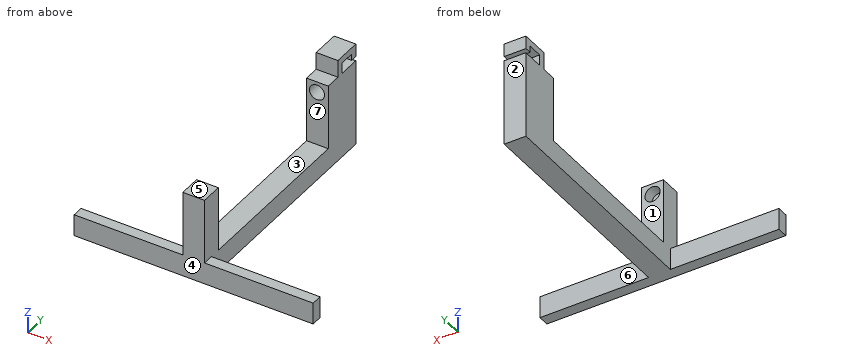
```python
from build123d import *

# Parameters (mm, degrees)
SKICA1_W                      = 10
SKICA1_H                      = 10
P_IDAT_VYSUNUT_M1_DEPTH       = 10
SKICA2_R                      = 3.5
ODEBRAT_VYSUNUT_M1_DEPTH      = 5
SKICA6_W                      = 10
SKICA6_H                      = 10
P_IDAT_VYSUNUT_M9_DEPTH       = 30
SKICA7_W                      = 10
SKICA7_H                      = 10
P_IDAT_VYSUNUT_M11_DEPTH      = 100
SKICA8_W                      = 10
SKICA8_H                      = 10
P_IDAT_VYSUNUT_M12_DEPTH      = 30
SKICA9_W                      = 10
SKICA9_H                      = 10
P_IDAT_VYSUNUT_M13_DEPTH      = 10
SKICA10_R                     = 3.5
ODEBRAT_VYSUNUT_M2_DEPTH      = 10
SKICA20_W                     = 10
SKICA20_H                     = 10
P_IDAT_VYSUNUT_M21_DEPTH      = 20
P_IDAT_VYSUNUT_M22_DEPTH      = 50
P_IDAT_VYSUNUT_M22_DEPTH_BACK = 60
SKICA11_W                     = 10
SKICA11_H                     = 5
SKICA10_2_R                   = 3.5
ODEBRAT_VYSUNUT_M7_DEPTH      = 15
SKICA21_W                     = 10
SKICA21_H                     = 3
P_IDAT_VYSUNUT_M24_DEPTH      = 8
SKICA22_W                     = 10
SKICA22_H                     = 3
P_IDAT_VYSUNUT_M25_DEPTH      = 10
SKICA23_W                     = 10
SKICA23_H                     = 3
P_IDAT_VYSUNUT_M26_DEPTH      = 3


with BuildPart() as part:
    # Skica1 → P_idat vysunut_m1 (new body)
    with BuildSketch(Plane.XY):
        with Locations((5, 5)):
            Rectangle(SKICA1_W, SKICA1_H)
    extrude(amount=P_IDAT_VYSUNUT_M1_DEPTH)

    # Skica2 → Odebrat vysunut_m1 (cut)
    with BuildSketch(Plane(origin=(0, 10, 0), x_dir=(1, 0, 0), z_dir=(0, 1, 0))):
        with Locations(Location((5, -5, 0), (0, 0, 270))):
            Circle(SKICA2_R)
    extrude(amount=-ODEBRAT_VYSUNUT_M1_DEPTH, mode=Mode.SUBTRACT)

    # Skica6 → P_idat vysunut_m9 (add)
    with BuildSketch(Plane(origin=(0, 0, 0), x_dir=(-1, 0, 0), z_dir=(0, 0, -1))):
        with Locations((-5, 5)):
            Rectangle(SKICA6_W, SKICA6_H)
    extrude(amount=P_IDAT_VYSUNUT_M9_DEPTH)

    # Skica7 → P_idat vysunut_m11 (add)
    with BuildSketch(Plane(origin=(0, 10, 0), x_dir=(1, 0, 0), z_dir=(0, 1, 0))):
        with Locations((5, 25)):
            Rectangle(SKICA7_W, SKICA7_H)
    extrude(amount=P_IDAT_VYSUNUT_M11_DEPTH)

    # Skica8 → P_idat vysunut_m12 (add)
    with BuildSketch(Plane.XY.offset(-20)):
        with Locations((5, 105)):
            Rectangle(SKICA8_W, SKICA8_H)
    extrude(amount=P_IDAT_VYSUNUT_M12_DEPTH)

    # Skica9 → P_idat vysunut_m13 (add)
    with BuildSketch(Plane.XZ.offset(-100)):
        with Locations((5, 5)):
            Rectangle(SKICA9_W, SKICA9_H)
    extrude(amount=P_IDAT_VYSUNUT_M13_DEPTH)

    # Skica10 → Odebrat vysunut_m2 (cut)
    with BuildSketch(Plane.XZ.offset(-90)):
        with Locations(Location((4.797944497, 5, 0), (0, 0, 270))):
            Circle(SKICA10_R)
    extrude(amount=-ODEBRAT_VYSUNUT_M2_DEPTH, mode=Mode.SUBTRACT)

    # Skica20 → P_idat vysunut_m21 (add)
    with BuildSketch(Plane(origin=(0, 0, 0), x_dir=(-1, 0, 0), z_dir=(0, 0, -1))):
        with Locations((-5, 95)):
            Rectangle(SKICA20_W, SKICA20_H)
    extrude(amount=P_IDAT_VYSUNUT_M21_DEPTH)

    # Skica11 → P_idat vysunut_m22 (add, two sides: drawn at the far end of the back side and taken through both)
    with BuildSketch(Plane(origin=(10, 0, 0), x_dir=(0, 0, -1), z_dir=(1, 0, 0)).offset(-P_IDAT_VYSUNUT_M22_DEPTH_BACK)):
        with Locations((25, 2.5)):
            Rectangle(SKICA11_W, SKICA11_H)
    extrude(amount=P_IDAT_VYSUNUT_M22_DEPTH + P_IDAT_VYSUNUT_M22_DEPTH_BACK)

    # Skica10_2 → Odebrat vysunut_m7 (cut)
    with BuildSketch(Plane.XZ.offset(-90)):
        with Locations(Location((4.797944497, 5, 0), (0, 0, 270))):
            Circle(SKICA10_2_R)
    extrude(amount=-ODEBRAT_VYSUNUT_M7_DEPTH, mode=Mode.SUBTRACT)

    # Skica21 → P_idat vysunut_m24 (add)
    with BuildSketch(Plane.XY.offset(10)):
        with Locations((5, 98.5)):
            Rectangle(SKICA21_W, SKICA21_H)
    extrude(amount=P_IDAT_VYSUNUT_M24_DEPTH)

    # Skica22 → P_idat vysunut_m25 (add)
    with BuildSketch(Plane(origin=(0, 100, 0), x_dir=(1, 0, 0), z_dir=(0, 1, 0))):
        with Locations((5, -16.5)):
            Rectangle(SKICA22_W, SKICA22_H)
    extrude(amount=P_IDAT_VYSUNUT_M25_DEPTH)

    # Skica23 → P_idat vysunut_m26 (add)
    with BuildSketch(Plane(origin=(0, 0, 15), x_dir=(-1, 0, 0), z_dir=(0, 0, -1))):
        with Locations((-5, 108.5)):
            Rectangle(SKICA23_W, SKICA23_H)
    extrude(amount=P_IDAT_VYSUNUT_M26_DEPTH)


solid = part.part
```
The model under review builds one solid part; all positions refer to its coordinate system, in mm. Face numbers are marked on the shaded views. A direction names the side the tool comes from. Coordinates: 2 decimals unless noted, no trailing zeros. Write each loop counter-clockwise with the first axis right and the second up, starting at its lowest first coordinate (ties: lowest second). Pieces come first, ordered by that corner, then holes. Notation, with made-up numbers: (44.25, -3) - (85.25, -3) arc R30 cw to (85.25, 28) - close; hole circle Ø4 at (27, 83). An arc over 180 degrees is marked (long way). Answer in a Markdown table with one row per item. Add a question column.
Q1. For the marked faces 5, 6 and 7, list the 3-axis set-ups (+Z, -Z, +X, -X, +Y, -Y) from which the entire face can be reached by the end or side of a thin tool; tool diameter is ignored.
Q2. Consider section D-D on y = 58. Give the boundary of the cut face in (x, z), then the cut area to 3 significant figures.
Q3. Clearance check with flat-ended pins moving along their axes: pin 1 (4 mm diameter, centred on x = 5, z = 5, fed in from -Y); pin 2 (5 mm diameter, centred on x = -20, z = -22.5, fed in from +Y); pin 3 (0.9 mm diameter, centred on x = 2.5, z = 13.5, fed in from -Y); pin 4 (2.5 mm diameter, centred on x = 43.5, y = 3, fed in from +Z). State where each tip first meets the part, or that it passes through.
Q4. Consider section C-C on z = 5. Give the boundary of the cut face in (x, y), then the cut area to 3 significant figures.
Q5. Consider section B-B on x = -30. Give the boundary of the cut face in (y, z), then the cut area to 3 significant figures.
Q6. Draft analysis for pull direction Y (two halves, no side actions). For the marked faces 1, 2, 3 and 4, state which applies: +Y half, -Y half, draft (parallel to the pull), parting line (faces both ways), or undercut.
Q7. Consider section A-A on z = -18. Give the boundary of the cut face in (x, y), then the cut area to 3 significant figures.
Q8. To check wall thickness, follow line 1 along X through (y, z) = (97, 5); line 2 along X through (y, z) = (8.35, 5); line 3 along Y through (x, z) = (7.5, 6.5). State the ranges of each line that lie inside material, in increasing order. Write a range as from..to.
Answers below:
| question | item | result |
|---|---|---|
| 1 | face 5 | +Z, +X, -X, -Y |
| 1 | face 6 | +Z, -Z, +X, +Y |
| 1 | face 7 | +Z, +X, -X |
| 2 | outline | (0, -30) - (10, -30) - (10, -20) - (0, -20) - close |
| 2 | area | 100 mm² |
| 3 | pin 1 | y = 0 |
| 3 | pin 2 | y = 5 |
| 3 | pin 3 | y = 97 |
| 3 | pin 4 | z = -20 |
| 4 | outline | (0, 0) - (10, 0) - (10, 10) - (8.5, 10) - (8.5, 5) - (1.5, 5) - (1.5, 10) - (0, 10) - close; (0, 90) - (1.3, 90) - (1.3, 105) - (8.3, 105) - (8.3, 90) - (10, 90) - (10, 110) - (0, 110) - close |
| 4 | area | 160 mm² |
| 5 | outline | (0, -30) - (5, -30) - (5, -20) - (0, -20) - close |
| 5 | area | 50.0 mm² |
| 6 | face 1 | undercut |
| 6 | face 2 | +Y half |
| 6 | face 3 | undercut |
| 6 | face 4 | -Y half |
| 7 | outline | (0, 0) - (10, 0) - (10, 10) - (0, 10) - close; (0, 90) - (10, 90) - (10, 110) - (0, 110) - close |
| 7 | area | 300 mm² |
| 8 | line 1 | 0..1.3, 8.3..10 |
| 8 | line 2 | 0..1.5, 8.5..10 |
| 8 | line 3 | 0..5, 105..110 |
